Can you work these out from the model? Positions are in its coordinate system, mm. Face numbers are marked on the shaded views. Give positions to 0.01 mm unless a question says otherwise; leave off trailing zeros. Write each loop counter-clockwise with the first axis right and the second up, starting at its lowest first coordinate (ties: lowest second). Pieces come first, ordered by that corner, then holes.
```python
from build123d import *

# Parameters (mm, degrees)
CYLINDER2014_R     = 59
CYLINDER2014_DEPTH = 16
CYLINDER2078_R     = 17
CYLINDER2078_DEPTH = 160
CYLINDER2021_R     = 4
CYLINDER2021_DEPTH = 100
CYLINDER2022_R     = 4
CYLINDER2022_DEPTH = 100
CYLINDER2042_R     = 1.5
CYLINDER2042_DEPTH = 100
CYLINDER2058_R     = 1.5
CYLINDER2058_DEPTH = 100
CYLINDER2057_R     = 1.5
CYLINDER2057_DEPTH = 100
CYLINDER2039_R     = 1.5
CYLINDER2039_DEPTH = 100
CYLINDER2038_R     = 1.5
CYLINDER2038_DEPTH = 100
CYLINDER2037_R     = 1.5
CYLINDER2037_DEPTH = 100
CYLINDER2036_R     = 1.5
CYLINDER2036_DEPTH = 100
CYLINDER2061_R     = 1.5
CYLINDER2061_DEPTH = 100
CYLINDER2059_R     = 4
CYLINDER2059_DEPTH = 100
CYLINDER2020_R     = 4
CYLINDER2020_DEPTH = 100
CYLINDER2019_R     = 4
CYLINDER2019_DEPTH = 100
CYLINDER2017_R     = 4
CYLINDER2017_DEPTH = 100
CYLINDER2015_R     = 4
CYLINDER2015_DEPTH = 100
CYLINDER2016_R     = 4
CYLINDER2016_DEPTH = 100
CYLINDER2018_R     = 4
CYLINDER2018_DEPTH = 100
CYLINDER2060_R     = 4
CYLINDER2060_DEPTH = 100
CYLINDER2029_R     = 4
CYLINDER2029_DEPTH = 20
CYLINDER2028_R     = 4
CYLINDER2028_DEPTH = 20
CYLINDER2027_R     = 4
CYLINDER2027_DEPTH = 20
CYLINDER2026_R     = 4
CYLINDER2026_DEPTH = 40
CYLINDER2025_R     = 4
CYLINDER2025_DEPTH = 40
CYLINDER2024_R     = 4
CYLINDER2024_DEPTH = 40
CYLINDER2023_R     = 4
CYLINDER2023_DEPTH = 40
CYLINDER2050_R     = 4
CYLINDER2050_DEPTH = 20
CYLINDER2030_R     = 59
CYLINDER2030_DEPTH = 16
CHAMFER071_SIZE    = 4
FILLET007_R        = 4


with BuildPart() as obj1:
    # Cylinder2014 → Cylinder2014 (new body)
    with BuildSketch(Plane(origin=(-0.5, 0, 19.85), x_dir=(1, 0, 0), z_dir=(0, 0, 1))):
        Circle(CYLINDER2014_R)
    extrude(amount=CYLINDER2014_DEPTH)


with BuildPart() as obj2:
    # Cylinder2078 → Cylinder2078 (new body)
    with BuildSketch(Plane(origin=(-18, 0, -60), x_dir=(1, 0, 0), z_dir=(0, 0, 1))):
        Circle(CYLINDER2078_R)
    extrude(amount=CYLINDER2078_DEPTH)


with BuildPart() as obj3:
    # Cylinder2021 → Cylinder2021 (new body)
    with BuildSketch(Plane(origin=(14, 0, -18), x_dir=(1, 0, 0), z_dir=(0, 0, 1))):
        Circle(CYLINDER2021_R)
    extrude(amount=CYLINDER2021_DEPTH)


with BuildPart() as obj4:
    # Cylinder2022 → Cylinder2022 (new body)
    with BuildSketch(Plane(origin=(90, 0, -18), x_dir=(1, 0, 0), z_dir=(0, 0, 1))):
        Circle(CYLINDER2022_R)
    extrude(amount=CYLINDER2022_DEPTH)

    # Compound1009: union obj3
    add(obj3.part)


with BuildPart() as obj5:
    # Cylinder2042 → Cylinder2042 (new body)
    with BuildSketch(Plane(origin=(-34, -16, -60), x_dir=(1, 0, 0), z_dir=(0, 0, 1))):
        Circle(CYLINDER2042_R)
    extrude(amount=CYLINDER2042_DEPTH)


with BuildPart() as obj6:
    # Cylinder2058 → Cylinder2058 (new body)
    with BuildSketch(Plane(origin=(34, -16, -60), x_dir=(1, 0, 0), z_dir=(0, 0, 1))):
        Circle(CYLINDER2058_R)
    extrude(amount=CYLINDER2058_DEPTH)


with BuildPart() as obj7:
    # Cylinder2057 → Cylinder2057 (new body)
    with BuildSketch(Plane(origin=(34, 16, -60), x_dir=(1, 0, 0), z_dir=(0, 0, 1))):
        Circle(CYLINDER2057_R)
    extrude(amount=CYLINDER2057_DEPTH)


with BuildPart() as obj8:
    # Cylinder2039 → Cylinder2039 (new body)
    with BuildSketch(Plane(origin=(16, 34, -60), x_dir=(1, 0, 0), z_dir=(0, 0, 1))):
        Circle(CYLINDER2039_R)
    extrude(amount=CYLINDER2039_DEPTH)


with BuildPart() as obj9:
    # Cylinder2038 → Cylinder2038 (new body)
    with BuildSketch(Plane(origin=(10, -36, -60), x_dir=(1, 0, 0), z_dir=(0, 0, 1))):
        Circle(CYLINDER2038_R)
    extrude(amount=CYLINDER2038_DEPTH)


with BuildPart() as obj10:
    # Cylinder2037 → Cylinder2037 (new body)
    with BuildSketch(Plane(origin=(-16, -34, -60), x_dir=(1, 0, 0), z_dir=(0, 0, 1))):
        Circle(CYLINDER2037_R)
    extrude(amount=CYLINDER2037_DEPTH)


with BuildPart() as obj11:
    # Cylinder2036 → Cylinder2036 (new body)
    with BuildSketch(Plane(origin=(-16, 34, -60), x_dir=(1, 0, 0), z_dir=(0, 0, 1))):
        Circle(CYLINDER2036_R)
    extrude(amount=CYLINDER2036_DEPTH)


with BuildPart() as obj12:
    # Cylinder2061 → Cylinder2061 (new body)
    with BuildSketch(Plane(origin=(-34, 16, -60), x_dir=(1, 0, 0), z_dir=(0, 0, 1))):
        Circle(CYLINDER2061_R)
    extrude(amount=CYLINDER2061_DEPTH)

    # Compound993: union obj5, obj6, obj7, obj8, obj9, obj10, obj11
    add(obj5.part)
    add(obj6.part)
    add(obj7.part)
    add(obj8.part)
    add(obj9.part)
    add(obj10.part)
    add(obj11.part)


with BuildPart() as obj13:
    # Cylinder2059 → Cylinder2059 (new body)
    with BuildSketch(Plane(origin=(-16, 34, -90), x_dir=(1, 0, 0), z_dir=(0, 0, 1))):
        Circle(CYLINDER2059_R)
    extrude(amount=CYLINDER2059_DEPTH)


with BuildPart() as obj14:
    # Cylinder2020 → Cylinder2020 (new body)
    with BuildSketch(Plane(origin=(-16, -34, -90), x_dir=(1, 0, 0), z_dir=(0, 0, 1))):
        Circle(CYLINDER2020_R)
    extrude(amount=CYLINDER2020_DEPTH)


with BuildPart() as obj15:
    # Cylinder2019 → Cylinder2019 (new body)
    with BuildSketch(Plane(origin=(34, -16, -90), x_dir=(1, 0, 0), z_dir=(0, 0, 1))):
        Circle(CYLINDER2019_R)
    extrude(amount=CYLINDER2019_DEPTH)


with BuildPart() as obj16:
    # Cylinder2017 → Cylinder2017 (new body)
    with BuildSketch(Plane(origin=(16, 34, -90), x_dir=(1, 0, 0), z_dir=(0, 0, 1))):
        Circle(CYLINDER2017_R)
    extrude(amount=CYLINDER2017_DEPTH)


with BuildPart() as obj17:
    # Cylinder2015 → Cylinder2015 (new body)
    with BuildSketch(Plane(origin=(10, -36, -90), x_dir=(1, 0, 0), z_dir=(0, 0, 1))):
        Circle(CYLINDER2015_R)
    extrude(amount=CYLINDER2015_DEPTH)


with BuildPart() as obj18:
    # Cylinder2016 → Cylinder2016 (new body)
    with BuildSketch(Plane(origin=(-34, 16, -90), x_dir=(1, 0, 0), z_dir=(0, 0, 1))):
        Circle(CYLINDER2016_R)
    extrude(amount=CYLINDER2016_DEPTH)


with BuildPart() as obj19:
    # Cylinder2018 → Cylinder2018 (new body)
    with BuildSketch(Plane(origin=(34, 16, -90), x_dir=(1, 0, 0), z_dir=(0, 0, 1))):
        Circle(CYLINDER2018_R)
    extrude(amount=CYLINDER2018_DEPTH)


with BuildPart() as obj20:
    # Cylinder2060 → Cylinder2060 (new body)
    with BuildSketch(Plane(origin=(-34, -16, -90), x_dir=(1, 0, 0), z_dir=(0, 0, 1))):
        Circle(CYLINDER2060_R)
    extrude(amount=CYLINDER2060_DEPTH)

    # Compound1008: union obj13, obj14, obj15, obj16, obj17, obj18, obj19
    add(obj13.part)
    add(obj14.part)
    add(obj15.part)
    add(obj16.part)
    add(obj17.part)
    add(obj18.part)
    add(obj19.part)


with BuildPart() as obj21:
    # Cylinder2029 → Cylinder2029 (new body)
    with BuildSketch(Plane(origin=(103, 12, -20), x_dir=(1, 0, 0), z_dir=(0, 0, 1))):
        Circle(CYLINDER2029_R)
    extrude(amount=CYLINDER2029_DEPTH)


with BuildPart() as obj22:
    # Cylinder2028 → Cylinder2028 (new body)
    with BuildSketch(Plane(origin=(76, 24, -18), x_dir=(1, 0, 0), z_dir=(0, 0, 1))):
        Circle(CYLINDER2028_R)
    extrude(amount=CYLINDER2028_DEPTH)


with BuildPart() as obj23:
    # Cylinder2027 → Cylinder2027 (new body)
    with BuildSketch(Plane(origin=(91, -27, -18), x_dir=(1, 0, 0), z_dir=(0, 0, 1))):
        Circle(CYLINDER2027_R)
    extrude(amount=CYLINDER2027_DEPTH)


with BuildPart() as obj24:
    # Cylinder2026 → Cylinder2026 (new body)
    with BuildSketch(Plane(origin=(13, -27, -18), x_dir=(1, 0, 0), z_dir=(0, 0, 1))):
        Circle(CYLINDER2026_R)
    extrude(amount=CYLINDER2026_DEPTH)


with BuildPart() as obj25:
    # Cylinder2025 → Cylinder2025 (new body)
    with BuildSketch(Plane(origin=(28, 24, -18), x_dir=(1, 0, 0), z_dir=(0, 0, 1))):
        Circle(CYLINDER2025_R)
    extrude(amount=CYLINDER2025_DEPTH)


with BuildPart() as obj26:
    # Cylinder2024 → Cylinder2024 (new body)
    with BuildSketch(Plane(origin=(1, -12, -18), x_dir=(1, 0, 0), z_dir=(0, 0, 1))):
        Circle(CYLINDER2024_R)
    extrude(amount=CYLINDER2024_DEPTH)


with BuildPart() as obj27:
    # Cylinder2023 → Cylinder2023 (new body)
    with BuildSketch(Plane(origin=(1, 12, -18), x_dir=(1, 0, 0), z_dir=(0, 0, 1))):
        Circle(CYLINDER2023_R)
    extrude(amount=CYLINDER2023_DEPTH)


with BuildPart() as obj28:
    # Cylinder2050 → Cylinder2050 (new body)
    with BuildSketch(Plane(origin=(103, -12, -20), x_dir=(1, 0, 0), z_dir=(0, 0, 1))):
        Circle(CYLINDER2050_R)
    extrude(amount=CYLINDER2050_DEPTH)

    # Compound1007: union obj21, obj22, obj23, obj24, obj25, obj26, obj27
    add(obj21.part)
    add(obj22.part)
    add(obj23.part)
    add(obj24.part)
    add(obj25.part)
    add(obj26.part)
    add(obj27.part)


with BuildPart() as common003:
    # Cylinder2030 → Cylinder2030 (new body)
    with BuildSketch(Plane.XY.offset(2)):
        Circle(CYLINDER2030_R)
    extrude(amount=CYLINDER2030_DEPTH)

    # Cut669: cut obj28
    add(obj28.part, mode=Mode.SUBTRACT)

    # Cut670: cut obj20
    add(obj20.part, mode=Mode.SUBTRACT)

    # Cut674: cut obj12
    add(obj12.part, mode=Mode.SUBTRACT)

    # Chamfer071
    chamfer071_edges = [common003.edges().sort_by_distance(p)[0] for p in [
        (-59, 0, 2),
    ]]
    chamfer(chamfer071_edges, length=CHAMFER071_SIZE)

    # Cut675: cut obj4
    add(obj4.part, mode=Mode.SUBTRACT)


with BuildPart() as common003_1:
    # Cut675 placement: moved
    add(common003.part.moved(Location((-0.5, 0, 14))))

    # Cut668: cut obj2
    add(obj2.part, mode=Mode.SUBTRACT)

    # Fillet007
    fillet007_edges = [common003_1.edges().sort_by_distance(p)[0] for p in [
        (-35, 0, 32),
    ]]
    fillet(fillet007_edges, radius=FILLET007_R)


with BuildPart() as common003_2:
    # Fillet007 placement: moved
    add(common003_1.part.moved(Location((0, 0, -0.15))))

    # Common003: intersect obj1
    add(obj1.part, mode=Mode.INTERSECT)


solid = common003_2.part
```
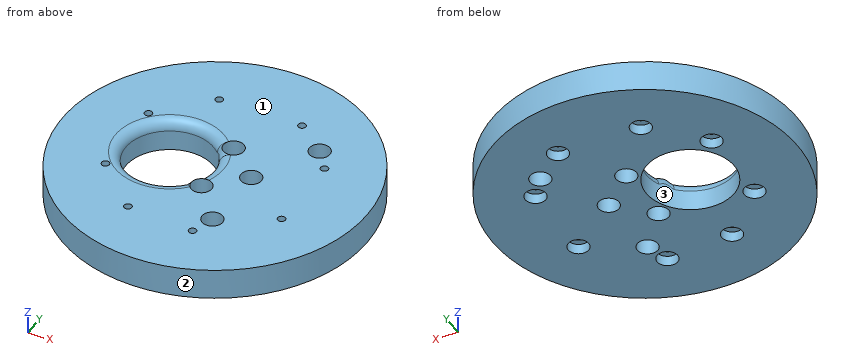
1) Please list where these lines run through material, in increasing order: L1, parallel to X at y = 0.5, z = 23.5; L2, parallel to X at y = -1, z = 29.75; L3, parallel to Y at x = 33.5, z = 29.25.
Values follow:
L1: x = -59.5 to -34.99, -1.01 to 9.53, 17.47 to 58.5
L2: x = -59.49 to -35.45, -0.55 to 9.63, 17.37 to 58.49
L3: y = -48.22 to -17.5, -14.5 to 14.5, 17.5 to 48.22
2) Suppose I cut it at A-A on z = 22. State how many separate pieces and enclosed holes the cut face has, plus the area to 3 significant figures.
Values follow:
separate pieces: 1
enclosed holes: 14
area: 9,370 mm2
3) Suppose I cut it at C-C on x = 27.5. Write out the boundary of the cut face in (y, z).
Values follow:
outline: (-51.93, 19.85) - (20, 19.85) - (20, 31.85) - (-51.93, 31.85) - close; (28, 19.85) - (51.93, 19.85) - (51.93, 31.85) - (28, 31.85) - close
4) Suppose I cut it at B-B on y = 0. Write out the boundary of the cut face in (x, z).
Values follow:
outline: (-59.5, 19.85) - (-35, 19.85) - (-35, 27.85) arc R4 ccw to (-39, 31.85) - (-59.5, 31.85) - close; (-1, 19.85) - (9.5, 19.85) - (9.5, 31.85) - (3, 31.85) arc R4 ccw to (-1, 27.85) - close; (17.5, 19.85) - (58.5, 19.85) - (58.5, 31.85) - (17.5, 31.85) - close
5) Suppose I cut it at D-D on y = -28.5. Write out the boundary of the cut face in (x, z), plus the area to 3 significant figures.
Values follow:
outline: (-52.16, 19.85) - (8.79, 19.85) - (8.79, 31.85) - (-52.16, 31.85) - close; (16.21, 19.85) - (51.16, 19.85) - (51.16, 31.85) - (16.21, 31.85) - close
area: 1,150 mm2
6) If we mould it in two halves opening along X, with no side actions, what happens to the marked faces 1, 2 and 3? For each: +X half, -X half, draft (parallel to the pull), parting line (faces both ways), or undercut.
Values follow:
face 1: draft
face 2: parting line
face 3: undercut
7) For pin 1 Ø2.5 at (x, y) = (-33.5, 14) entering from -Z; pin 2 Ø20.5 at (x, y) = (-18, 0) entering from +Z; pin 3 Ø6 at (x, z) = (-6.5, 22) entering from +Y; pin 4 Ø4 at (x, z) = (-26, 21.5) entering from +Y, each with a flat end and sliding along its axis, tell me the tip position at first contact or that it passes through.
Values follow:
pin 1: stops at z = 23.85
pin 2: passes through
pin 3: stops at y = 58.92
pin 4: stops at y = 54.12
